Here's how the part is built. I have some questions about the finished solid (model axes, mm). Round coordinates to 2 decimals unless told otherwise and drop trailing zeros. Write each loop counter-clockwise with the first axis right and the second up, starting at its lowest first coordinate (ties: lowest second). Pieces come first, ordered by that corner, then holes. Notation, with made-up numbers: (-1, 74) -> (48, 74) arc R24 ccw to (48, 86) -> close; hole circle Ø11 at (49, 33.5). An arc over 180 degrees is marked (long way). Put each result on its own line as item: value. Start each with the question number.
1. Suppose I cut it at B-B (y = 6.5). Count the separate pieces of the cut face and the enclosed holes in it, then the cut area to 3 significant figures.
2. We'd pull the mould along Z, two halves only. Please class faces 1 (the face through (20.8, 5.37, 11.97)), 2 (the face through (-15.4, 5.37, 18.41)), 3 (the face through (4, 0, 23)): +Z half, -Z half, draft (parallel to the pull), parting line (faces both ways), or undercut.
3. Suppose I cut it at A-A (x = -16). Please give me the cut outline in (y, z).
4. For pin 1 (3 mm diameter, centred on y = 8.5, z = 8.5, fed in from +X); pin 2 (1 mm diameter, centred on x = 2.5, y = 3.5, fed in from +Z); pin 3 (4 mm diameter, centred on y = 1.5, z = 0, fed in from -X), each with a flat end and sliding along its axis, tell me the tip position at first contact or that it passes through.
5. Suppose I cut it at C-C (x = -27). Please give me the cut outline in (y, z), then the cut area to 3 significant figures.
6. I need wall thicknesses on probe 1 along Z at (x, y) = (13.5, 2.5); probe 2 along Z at (x, y) = (-14.5, 8.5); probe 3 along X at (y, z) = (8.5, -1.5). Which ranges of each line are inside material? Lowest first, please. Write a range as from..to.
```python
from build123d import *

# Parameters (mm, degrees)
SKETCH1_W            = 6
SKETCH1_H            = 10.6
BOSS_EXTRUDE1_DEPTH  = 10.6
CIRPATTERN2_COUNT    = 18
M3_CLEARANCE_HOLE1_D = 3.4
CIRPATTERN1_COUNT    = 6


with BuildPart() as part:
    # Sketch1 → Revolve1 (revolve)
    with BuildSketch(Plane.XY, mode=Mode.PRIVATE) as revolve1_sk:
        with Locations((27, 5.3)):
            Rectangle(SKETCH1_W, SKETCH1_H)
    revolve(revolve1_sk.sketch.rotate(Axis((0, 22.026442308, 0), (0, -1, 0)), 180), axis=Axis((0, 22.026442308, 0), (0, -1, 0)))

    # Sketch4 → Boss-Extrude1 (add)
    with BuildSketch(Plane(origin=(0, 10.6, 0), x_dir=(1, 0, 0), z_dir=(0, 1, 0))):
        with BuildLine():
            Line((22.771936798, 0.68551001), (29.077470181, 7.382460828))
            ThreePointArc((29.077470181, 7.382460828), (30, 0), (29.077470181, -7.382460828))
            Line((29.077470181, -7.382460828), (22.771936798, -0.68551001))
            ThreePointArc((22.771936798, -0.68551001), (22.5, 0), (22.771936798, 0.68551001))
        make_face()
    boss_extrude1 = extrude(amount=-BOSS_EXTRUDE1_DEPTH)

    # CirPattern2: Boss-Extrude1 ×18 about axis
    cirpattern2_axis = Axis((0, 0, 0), (0, 1, 0))
    for i in range(1, CIRPATTERN2_COUNT):
        add(boss_extrude1.rotate(cirpattern2_axis, i * 360 / CIRPATTERN2_COUNT))

    # M3 Clearance Hole1 (through all)
    with Locations(Plane(origin=(0, 10.6, 0), x_dir=(1, 0, 0), z_dir=(0, 1, 0))):
        with Locations((27, 0)):
            m3_clearance_hole1 = Hole(M3_CLEARANCE_HOLE1_D / 2)

    # CirPattern1: M3 Clearance Hole1 ×6 about axis
    cirpattern1_axis = Axis((0, 0, 0), (0, 1, 0))
    for i in range(1, CIRPATTERN1_COUNT):
        add(m3_clearance_hole1.rotate(cirpattern1_axis, i * 360 / CIRPATTERN1_COUNT), mode=Mode.SUBTRACT)


solid = part.part
```
Verdict:
1. separate pieces: 1
1. enclosed holes: 7
1. area: 1,030 mm^2
2. face 1: undercut
2. face 2: undercut
2. face 3: draft
3. outline: (0, -25.38) -> (10.6, -25.38) -> (10.6, -17.89) -> (0, -17.89) -> close; (0, 17.89) -> (10.6, 17.89) -> (10.6, 25.38) -> (0, 25.38) -> close
4. pin 1: stops at x = 29.17
4. pin 2: stops at z = 29.93
4. pin 3: stops at x = -30
5. outline: (0, -13.08) -> (10.6, -13.08) -> (10.6, -1.7) -> (0, -1.7) -> close; (0, 1.7) -> (10.6, 1.7) -> (10.6, 13.08) -> (0, 13.08) -> close
5. area: 241 mm^2
6. probe 1: z = -26.79..-25.08, -21.68..-19.74, 19.74..21.68, 25.08..26.79
6. probe 2: z = -26.26..-24.76, -22.01..-19.12, 19.12..22.01, 24.76..26.26
6. probe 3: x = -29.96..-27.8, -26.2..-23.54, 23.54..26.2, 27.8..29.96
